from build123d import *

# Parameters (mm, degrees)
SALIENTE_EXTRUIR1_DEPTH = 223.76
REDONDEO2_R             = 5


with BuildPart() as part:
    # Croquis1 → Saliente-Extruir1 (new body)
    with BuildSketch(Plane.XY):
        Polygon((11, 19), (15, 19), (15, 29), (-15, 29), (-15, -29), (15, -29), (15, -19), (11, -19), (11, -25), (-11, -25), (-11, 25), (11, 25), align=None)
    extrude(amount=-SALIENTE_EXTRUIR1_DEPTH)

    # Redondeo2
    redondeo2_edges = [part.edges().sort_by_distance(p)[0] for p in [
        (-15, 29, -111.88),
        (-15, -29, -111.88),
    ]]
    fillet(redondeo2_edges, radius=REDONDEO2_R)


solid = part.part
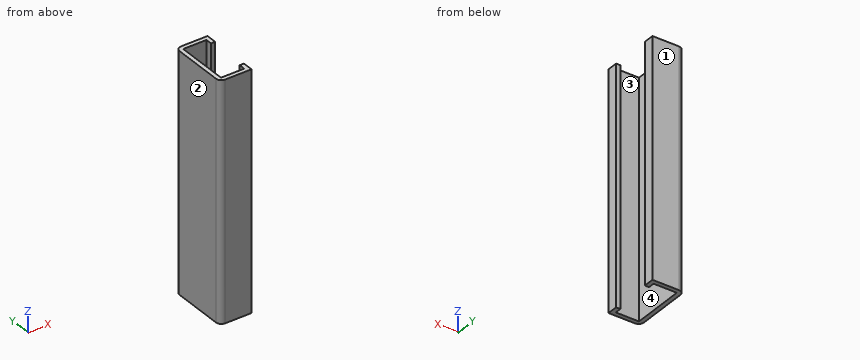
Geometry check sheet. Reference: the model listing, model coordinates, mm. Face numbers are marked on the shaded views. Round coordinates to 2 decimals unless told otherwise and drop trailing zeros. Order: outer loops, then holes, each group sorted by start corner. A loop starts at its lowest first (then second) coordinate and runs counter-clockwise, first axis right, second up. Notation, with made-up numbers: M 72,56 L 91,56 A34 ccw 91,88 Z; hole C 38,-18.75 d11. An arc over 180 degrees is marked long. Write each question's results on one line, items separated by ' | '. Start each with the question number.
1. Cross-section at A-A on x = 4.75. Record the boundary of the cut face in (y, z), plus the area to 3 significant figures.
2. Cross-section at C-C on y = -2. Record the boundary of the cut face in (x, z), plus the area to 3 significant figures.
3. Material ranges on L1, parallel to X at y = -20, z = -130.5; L2, parallel to Y at x = -2.5, z = -171; L3, parallel to X at y = 13.5, z = -166, recorded low to high. Write a range as from..to.
4. Go/stop test with a flat-tipped pin: P1, Ø5, axis at y = 6, z = -185, coming from the +X side. Record where the tip stops, or that it passes through.
5. Draft check along Y on the marked faces 1, 2, 3 and 4. Enter one of: pulls with the +Y half, pulls with the -Y half, needs draft (parallel to the pull), parting line crosses it, or undercut.
6. Cross-section at B-B on z = -196. Record the boundary of the cut face in (x, y), plus the area to 3 significant figures.
Resolved:
1) outline: M -29,-223.76 L -25,-223.76 L -25,0 L -29,0 Z; M 25,-223.76 L 29,-223.76 L 29,0 L 25,0 Z | area: 1,790 mm2
2) outline: M -15,-223.76 L -11,-223.76 L -11,0 L -15,0 Z | area: 895 mm2
3) L1: -15..-11, 11..15 | L2: -29..-25, 25..29 | L3: -15..-11
4) P1: x = -11
5) face 1: pulls with the +Y half | face 2: needs draft | face 3: undercut | face 4: undercut
6) outline: M -15,-24 A5 ccw -10,-29 L 15,-29 L 15,-19 L 11,-19 L 11,-25 L -11,-25 L -11,25 L 11,25 L 11,19 L 15,19 L 15,29 L -10,29 A5 ccw -15,24 Z | area: 477 mm2
